For this review, take the finished solid that the model builds, in its own axes (mm). Face numbers are marked on the shaded views. A direction names the side the tool comes from. Coordinates: 2 decimals unless noted, no trailing zeros. Write each loop counter-clockwise with the first axis right and the second up, starting at its lowest first coordinate (ties: lowest second). Pieces come first, ordered by that corner, then holes. Notation, with made-up numbers: M 33.5,-0.75 L 50.5,-0.75 A10 cw 50.5,17.25 Z; hole C 81.5,-39 d3. An arc over 180 degrees is marked long. One line per question, with ' | ' between items.
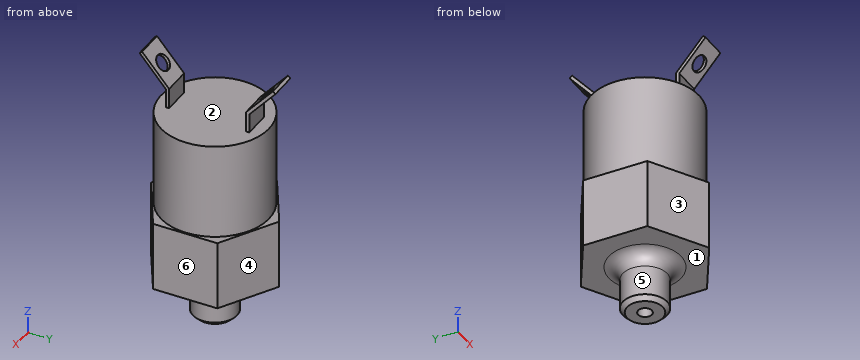
Autodesk Inventor part; units mm, degrees
ref_plane "YZ Plane" through (0, 0, 0) normal (1, 0, 0) x (0, 1, 0)
ref_plane "XZ Plane" through (0, 0, 0) normal (0, 1, 0) x (-1, 0, 0)
ref_plane "XY Plane" through (0, 0, 0) normal (0, 0, 1) x (1, 0, 0)
sketch "Sketch1" plane through (0, 0, 0) normal (0, 0, 1) x (1, 0, 0)
  line L0 (0, 14.6647) -> (12.7, 7.3323)
  line L1 (12.7, 7.3323) -> (12.7, -7.3323)
  line L2 (12.7, -7.3323) -> (0, -14.6647)
  line L3 (0, -14.6647) -> (-12.7, -7.3323)
  line L4 (-12.7, -7.3323) -> (-12.7, 7.3323)
  line L5 (-12.7, 7.3323) -> (0, 14.6647)
  line L6 (0, 14.6647) -> (0, 0)
  dimension "d0" = 25.4
extrude "Extrusion1" add sketch "Sketch1" along normal blind 15.875
sketch "Sketch2" plane through (0, 0, 0) normal (0, 0, -1) x (-1, 0, 0)
  line L0 (12.7, -7.3323) -> (12.7, 7.3323)
  line L1 (12.7, 7.3323) -> (0, 14.6647)
  line L2 (0, 14.6647) -> (-12.7, 7.3323)
  line L3 (-12.7, 7.3323) -> (-12.7, -7.3323)
  line L4 (-12.7, -7.3323) -> (0, -14.6647)
  line L5 (0, -14.6647) -> (12.7, -7.3323)
  line L6 (-6.35, 10.9985) -> (6.35, -10.9985) construction
  circle A0 centre (0, 0) radius 5.08
  dimension "d3" = 10.16
extrude "Extrusion2" add sketch "Sketch2" along normal blind 11.049 contours A0
sketch "Sketch3" plane through (0, 0, -11.049) normal (0, 0, -1) x (-1, 0, 0)
  circle A0 centre (0, 0) radius 5.08
  circle A1 centre (0, 0) radius 1.5875
  dimension "d6" = 3.175
extrude "Extrusion3" cut sketch "Sketch3" against normal blind 19.9898 contours A1
sketch "Sketch4" plane through (0, 0, 15.875) normal (0, 0, 1) x (1, 0, 0)
  line L0 (12.7, 7.3323) -> (12.7, -7.3323)
  line L1 (0, 14.6647) -> (12.7, 7.3323)
  line L2 (-12.7, 7.3323) -> (0, 14.6647)
  line L3 (-12.7, -7.3323) -> (-12.7, 7.3323)
  line L4 (0, -14.6647) -> (-12.7, -7.3323)
  line L5 (12.7, -7.3323) -> (0, -14.6647)
  line L6 (-6.35, 10.9985) -> (6.35, -10.9985)
  circle A0 centre (0, 0) radius 12.3825
  dimension "d9" = 24.765
extrude "Extrusion4" add sketch "Sketch4" along normal blind 21.971 contours A0 L6 | L6 A0
sketch "Sketch5" plane through (0, 0, 0) normal (1, 0, 0) x (0, 1, 0)
  line L0 (12.3825, 15.875) -> (12.3825, 37.846)
  line L1 (-12.3825, 37.846) -> (12.3825, 37.846)
  line L2 (-12.3825, 15.875) -> (12.3825, 15.875)
  line L3 (9.525, 37.846) -> (9.525, 42.2598)
  line L4 (9.525, 42.2598) -> (15.5086, 49.1328)
  line L5 (15.5086, 49.1328) -> (14.9339, 49.6332)
  line L6 (14.9339, 49.6332) -> (8.763, 42.545)
  line L7 (8.763, 42.545) -> (8.763, 37.846)
  line L8 (0, 37.846) -> (0, 32.3818)
  line L9 (-12.3825, 15.875) -> (-12.3825, 37.846)
  line L10 (12.3825, 37.846) -> (-12.3825, 37.846)
  line L11 (-9.525, 37.846) -> (-9.525, 42.2598)
  line L12 (-9.525, 42.2598) -> (-15.5086, 49.1328)
  line L13 (-15.5086, 49.1328) -> (-14.9339, 49.6332)
  line L14 (-14.9339, 49.6332) -> (-8.763, 42.545)
  line L15 (-8.763, 42.545) -> (-8.763, 37.846)
  dimension "d12" = 19.05
  dimension "d13" = 0.762
  dimension "d14" = 0.762
  dimension "d15" = 4.699
  dimension "d17" = 9.398
extrude "Extrusion5" add sketch "Sketch5" along normal mid plane 6.35 contours L1 L7 L6 L5 L4 L3 | L11 L12 L13 L14 L15 L1
sketch "Sketch6" plane through (-3.175, -8.763, 42.545) normal (0, 0.7542, 0.6566) x (1, 0, 0)
  line L0 (6.35, -9.398) -> (6.35, 0)
  line L1 (0, 0) -> (6.35, 0)
  line L2 (0, 0) -> (0, -9.398)
  line L3 (0, -9.398) -> (6.35, -9.398)
  circle A0 centre (3.175, -4.699) radius 1.8713
extrude "Extrusion6" cut sketch "Sketch6" against normal blind 6.35 contours A0
mirror "Mirror1" about plane through (0, 0, 0) normal (0, 1, 0) of "Extrusion6"
thread "Thread1"
chamfer "Chamfer1" distance 1 angle 45 1 edges at (5.08, 0, -11.049)
fillet "Fillet1" radius 3.175 1 edges at (5.08, 0, 0)
equation "\"d14\" = d13"
properties part number "SM-2B-115R"
1. Take a section at D-D on z = 15. State the section outline as (x, y) points, plus the area to 3 significant figures.
Computed values:
outline: M -12.7,-7.33 L 0,-14.66 L 12.7,-7.33 L 12.7,7.33 L 0,14.66 L -12.7,7.33 Z | area: 559 mm2
2. Draft analysis for pull direction Y (two halves, no side actions). For the marked faces 1, 2, 3 and 4, state which applies: pulls with the +Y half, pulls with the -Y half, needs draft (parallel to the pull), parting line crosses it, or undercut.
Computed values:
face 1: needs draft | face 2: undercut | face 3: pulls with the -Y half | face 4: pulls with the +Y half
3. For line 1 along Y through (x, z) = (0, 0.25); line 2 along Z through (x, y) = (-3.5, 8); line 3 along Z through (x, y) = (3.5, -1.5), list the stretches that pass through material, from the lowest coordinate up.
Computed values:
line 1: y = -14.66 to -1.59, 1.59 to 14.66 | line 2: z = 0 to 37.85 | line 3: z = -11.05 to 37.85
4. Take a section at A-A on z = 5. State the section outline as (x, y) points (1 decimal).
Computed values:
outline: M -12.7,-7.3 L 0,-14.7 L 12.7,-7.3 L 12.7,7.3 L 0,14.7 L -12.7,7.3 Z; hole C 0,0 d3.2
5. Clearance check with flat-ended pins moving along their axes: P1, Ø4, axis at x = -8.5, y = 3, coming from the -Z side; P2, Ø2, axis at y = -12, z = 43.5, coming from the -X side; P3, Ø1.4, axis at x = -1, z = 39, coming from the -Y side (3 decimals); P4, Ø6, axis at x = -0.5, z = -1, coming from the +Y side. State where each tip first meets the part, or that it passes through.
Computed values:
P1: stops at z = -0.25 | P2: passes through | P3: stops at y = -9.525 | P4: stops at y = 14.66
6. Machinability: for the marked faces 5 and 6, which of the approach directions +Z, -Z, +X, -X, +Y, -Y give a long, thin tool a straight path to every point of the face, cutting with its end or side? Answer none if there is none.
Computed values:
face 5: -Z | face 6: +Z, -Z, +X, +Y, -Y
7. Take a section at C-C on x = -9. State the section outline as (y, z) points (3 decimals).
Computed values:
outline: M -9.469,0 L 9.469,0 L 9.469,15.875 L 8.504,15.875 L 8.504,37.846 L -8.504,37.846 L -8.504,15.875 L -9.469,15.875 Z
